```python
from build123d import *

# Parameters (mm, degrees)
SKETCH1_W                      = 10
SKETCH1_H                      = 25
CUT_EXTRUDE1_DEPTH             = 37.742346142
CUT_EXTRUDE2_DEPTH             = 37.742346142
CUT_EXTRUDE3_DEPTH             = 37.742346142
CUT_EXTRUDE4_DEPTH             = 37.742346142
CUT_EXTRUDE5_DEPTH             = 37.742346142
BOSS_EXTRUDE1_DEPTH            = 1.5
F_25_0_25_DIAMETER_HOLE1_D     = 25
F_25_0_25_DIAMETER_HOLE1_DEPTH = 4


with BuildPart() as part:
    # Sketch1 → Revolve1 (revolve)
    with BuildSketch(Plane(origin=(0, 0, 0), x_dir=(-1, 0, 0), z_dir=(0, 0, -1)), mode=Mode.PRIVATE) as revolve1_sk:
        with Locations((0, 12.5)):
            Rectangle(SKETCH1_W, SKETCH1_H)
    revolve(revolve1_sk.sketch.rotate(Axis((5, 0, 0), (-1, 0, 0)), 270), axis=Axis((5, 0, 0), (-1, 0, 0)))

    # Sketch2 → Cut-Extrude1 (cut, through all)
    with BuildSketch(Plane.ZY.offset(5)):
        Polygon((0.803847577, 17), (2.196152423, 17.803847577), (3, 19.196152423), (3, 20.803847577), (2.196152423, 22.196152423), (0.803847577, 23), (-0.803847577, 23), (-2.196152423, 22.196152423), (-3, 20.803847577), (-3, 19.196152423), (-2.196152423, 17.803847577), (-0.803847577, 17), align=None)
    extrude(amount=-CUT_EXTRUDE1_DEPTH, mode=Mode.SUBTRACT)

    # Sketch3 → Cut-Extrude2 (cut, through all)
    with BuildSketch(Plane.ZY.offset(5)):
        Polygon((-13.338288046, -17.142135624), (-11.945983201, -16.338288046), (-11.142135624, -14.945983201), (-11.142135624, -13.338288046), (-11.945983201, -11.945983201), (-13.338288046, -11.142135624), (-14.945983201, -11.142135624), (-16.338288046, -11.945983201), (-17.142135624, -13.338288046), (-17.142135624, -14.945983201), (-16.338288046, -16.338288046), (-14.945983201, -17.142135624), align=None)
    extrude(amount=-CUT_EXTRUDE2_DEPTH, mode=Mode.SUBTRACT)

    # Sketch4 → Cut-Extrude3 (cut, through all)
    with BuildSketch(Plane.ZY.offset(5)):
        Polygon((14.945983201, -17.142135624), (16.338288046, -16.338288046), (17.142135624, -14.945983201), (17.142135624, -13.338288046), (16.338288046, -11.945983201), (14.945983201, -11.142135624), (13.338288046, -11.142135624), (11.945983201, -11.945983201), (11.142135624, -13.338288046), (11.142135624, -14.945983201), (11.945983201, -16.338288046), (13.338288046, -17.142135624), align=None)
    extrude(amount=-CUT_EXTRUDE3_DEPTH, mode=Mode.SUBTRACT)

    # Sketch5 → Cut-Extrude4 (cut, through all)
    with BuildSketch(Plane.ZY.offset(5)):
        Polygon((16.338288046, 11.945983201), (17.142135624, 13.338288046), (17.142135624, 14.945983201), (16.338288046, 16.338288046), (14.945983201, 17.142135624), (13.338288046, 17.142135624), (11.945983201, 16.338288046), (11.142135624, 14.945983201), (11.142135624, 13.338288046), (11.945983201, 11.945983201), (13.338288046, 11.142135624), (14.945983201, 11.142135624), align=None)
    extrude(amount=-CUT_EXTRUDE4_DEPTH, mode=Mode.SUBTRACT)

    # Sketch6 → Cut-Extrude5 (cut, through all)
    with BuildSketch(Plane(origin=(5, 0, 0), x_dir=(0, 0, -1), z_dir=(1, 0, 0))):
        Polygon((16.338288046, 11.945983201), (17.142135624, 13.338288046), (17.142135624, 14.945983201), (16.338288046, 16.338288046), (14.945983201, 17.142135624), (13.338288046, 17.142135624), (11.945983201, 16.338288046), (11.142135624, 14.945983201), (11.142135624, 13.338288046), (11.945983201, 11.945983201), (13.338288046, 11.142135624), (14.945983201, 11.142135624), align=None)
    extrude(amount=-CUT_EXTRUDE5_DEPTH, mode=Mode.SUBTRACT)

    # Sketch7 → Boss-Extrude1 (add)
    with BuildSketch(Plane.ZY.offset(5)):
        Polygon((8.233090996, -8.233090996), (5.285969807, -10.374299875), (1.821421064, -11.5), (-1.821421064, -11.5), (-5.285969807, -10.374299875), (-8.233090996, -8.233090996), (-10.374299875, -5.285969807), (-11.5, -1.821421064), (-11.5, 1.821421064), (-10.374299875, 5.285969807), (-8.233090996, 8.233090996), (-5.285969807, 10.374299875), (-1.821421064, 11.5), (1.821421064, 11.5), (5.285969807, 10.374299875), (8.233090996, 8.233090996), (10.374299875, 5.285969807), (11.5, 1.821421064), (11.5, -1.821421064), (10.374299875, -5.285969807), align=None)
    extrude(amount=BOSS_EXTRUDE1_DEPTH)

    # 25.0 _25_ Diameter Hole1
    with Locations(Plane(origin=(5, 0, 0), x_dir=(0, 0, -1), z_dir=(1, 0, 0))):
        with Locations((0, 0)):
            Hole(F_25_0_25_DIAMETER_HOLE1_D / 2, depth=F_25_0_25_DIAMETER_HOLE1_DEPTH)


solid = part.part
```
Could you check a few things on this model? Use its own coordinates, in mm. A direction names the side the tool comes from. Coordinates: 2 decimals unless noted, no trailing zeros. Loops run counter-clockwise (first coordinate to the right, second up) from the corner with the lowest first, then second, coordinate; pieces in that order, holes last.
1) Imagine slicing it at C-C (x = -4). State how many separate pieces and enclosed holes the cut face has, and give its area (3 significant figures).
Reported:
separate pieces: 1
enclosed holes: 5
area: 1,820 mm2
2) Which directions (+Z, -Z, +X, -X, +Y, -Y) give clear straight access to the entire face, cutting with the end or side of a thin tool? Please do faces 1 (the face through (0, 17.142, 14)), 2 (the face through (1, 0, 0)), 3 (the face through (-5.74, 9.32, 6.74)), 4 (the face through (-5.74, -3.529, 10.945)).
Reported:
face 1: +X, -X
face 2: +X
face 3: +Z, -X, +Y
face 4: +Z, -X, -Y
3) Imagine slicing it at B-B (y = 0). List the corners of the cut face in (x, z) for me.
Reported:
outline: (-6.5, -11.5) - (-5, -11.5) - (-5, -25) - (5, -25) - (5, -12.5) - (1, -12.5) - (1, 12.5) - (5, 12.5) - (5, 25) - (-5, 25) - (-5, 11.5) - (-6.5, 11.5) - close
4) Imagine slicing it at A-A (z = 0). List the corners of the cut face in (x, y) for me.
Reported:
outline: (-6.5, -11.5) - (-5, -11.5) - (-5, -25) - (5, -25) - (5, -12.5) - (1, -12.5) - (1, 12.5) - (5, 12.5) - (5, 17) - (-5, 17) - (-5, 11.5) - (-6.5, 11.5) - close; (-5, 23) - (5, 23) - (5, 25) - (-5, 25) - close
5) Will these pins go through, and if not, where does the flat tip stop? pin 1 Ø4 at (x, z) = (-1.5, 2.5) entering from +Y (3 decimals); pin 2 Ø4 at (x, y) = (2.5, -3.5) entering from +Z; pin 3 Ø12 at (y, z) = (-0.5, 19) entering from -X.
Reported:
pin 1: stops at y = 24.995
pin 2: stops at z = 24.95
pin 3: stops at x = -5
6) Thinking about a two-plate mould opening in Y: for faces 5 (the face through (-5.74, -9.32, -6.74)), 6 (the face through (-6.5, 0, 0)), 7 (the face through (-0.07, -15.65, -11.55)), which applies, released by +Y, released by -Y, zero draft, split by the parting line, or undercut?
Reported:
face 5: released by -Y
face 6: zero draft
face 7: undercut
7) Please list where these lines run through material, in increasing order: line 1 along Y through (x, z) = (3.05, 0); line 2 along X through (y, z) = (0.5, 4); line 3 along X through (y, z) = (-20.5, -9).
Reported:
line 1: y = -25 to -12.5, 12.5 to 17, 23 to 25
line 2: x = -6.5 to 1
line 3: x = -5 to 5
